Autodesk Inventor part; units mm, degrees
ref_plane "YZ Plane" through (0, 0, 0) normal (1, 0, 0) x (0, 1, 0)
ref_plane "XZ Plane" through (0, 0, 0) normal (0, 1, 0) x (-1, 0, 0)
ref_plane "XY Plane" through (0, 0, 0) normal (0, 0, 1) x (1, 0, 0)
sketch "Skizze1" plane through (0, 0, 0) normal (0, 0, 1) x (1, 0, 0)
  line L0 (-9.8619, 0) -> (59.1713, 0)
  line L1 (0, -1.8) -> (0, 10.8)
  line L2 (0, 0) -> (0, 9)
  line L3 (0, 9) -> (7, 9)
  line L4 (7, 9) -> (9.3094, 5)
  line L5 (9.3094, 5) -> (49.3094, 5)
  line L6 (49.3094, 5) -> (49.3094, 0)
  line L7 (49.3094, 0) -> (0, 0)
  dimension "d0" = 18
  dimension "d1" = 7
  dimension "d3" = 10
  dimension "d4" = 40
  dimension "d16" = 60
revolve "Umdrehung1" add sketch "Skizze1" angle 360 about axis through (-10, 0, 0) along (1, 0, 0)
chamfer "Fase1" distance 1 angle 45 1 edges at (49.3094, -5, 0)
chamfer "Fase2" distance 0.5 angle 45 1 edges at (0, -9, 0)
thread "Gewinde1"
sketch "Skizze2" plane through (0, 0, 0) normal (-1, 0, 0) x (0, 0, 1)
  spline S0 degree 3 poles (0.7512, 3.8741) (0.7506, 3.8768) (0.75, 3.8795) (0.7227, 3.995) (0.6691, 4.1023) (0.5302, 4.2738) (0.4382, 4.3487) (0.229, 4.4493) (0.1117, 4.475) (0, 4.475) knots 2.407009 2.407009 2.407009 2.407009 2.415407 2.415407 2.762565 2.762565 3.097556 3.097556 3.432546 3.432546 3.432546 3.432546
  spline S1 degree 3 poles (0, 4.475) (-0.1117, 4.475) (-0.229, 4.4493) (-0.4383, 4.3487) (-0.5302, 4.2739) (-0.6692, 4.1024) (-0.7228, 3.995) (-0.7501, 3.8795) (-0.7507, 3.8768) (-0.7514, 3.8741) knots 3.432546 3.432546 3.432546 3.432546 3.767537 3.767537 4.102528 4.102528 4.449685 4.449685 4.458083 4.458083 4.458083 4.458083
  spline S2 degree 3 poles (-0.7514, 3.8741) (-0.7825, 3.7367) (-0.83, 3.604) (-0.9596, 3.341) (-1.058, 3.1943) (-1.298, 2.9367) (-1.4398, 2.8257) (-1.7272, 2.6597) (-1.8942, 2.5924) (-2.2374, 2.5134) (-2.4136, 2.5016) (-2.7062, 2.5208) (-2.8448, 2.546) (-2.9794, 2.5877) knots 7.439135 7.439135 7.439135 7.439135 7.853901 7.853901 8.351764 8.351764 8.849626 8.849626 9.347489 9.347489 9.845351 9.845351 10.260117 10.260117 10.260117 10.260117
  spline S3 degree 3 poles (-2.9794, 2.5877) (-2.982, 2.5886) (-2.9847, 2.5894) (-3.0984, 2.6235) (-3.2181, 2.6307) (-3.4362, 2.5961) (-3.547, 2.5539) (-3.7387, 2.423) (-3.8196, 2.3342) (-3.8755, 2.2375) knots 2.407009 2.407009 2.407009 2.407009 2.415407 2.415407 2.762565 2.762565 3.097556 3.097556 3.432546 3.432546 3.432546 3.432546
  spline S4 degree 3 poles (-3.8755, 2.2375) (-3.9313, 2.1408) (-3.9677, 2.0263) (-3.9853, 1.7948) (-3.9664, 1.6777) (-3.8873, 1.4716) (-3.8212, 1.3716) (-3.7348, 1.2902) (-3.7328, 1.2882) (-3.7307, 1.2863) knots 3.432546 3.432546 3.432546 3.432546 3.767537 3.767537 4.102528 4.102528 4.449685 4.449685 4.458083 4.458083 4.458083 4.458083
  spline S5 degree 3 poles (-3.7307, 1.2863) (-3.6273, 1.1907) (-3.5361, 1.0832) (-3.3732, 0.8394) (-3.2953, 0.6809) (-3.1922, 0.3442) (-3.167, 0.1659) (-3.1669, -0.166) (-3.1921, -0.3443) (-3.2953, -0.681) (-3.3731, -0.8395) (-3.536, -1.0833) (-3.6272, -1.1908) (-3.7306, -1.2865) knots 7.439135 7.439135 7.439135 7.439135 7.853901 7.853901 8.351764 8.351764 8.849626 8.849626 9.347489 9.347489 9.845351 9.845351 10.260117 10.260117 10.260117 10.260117
  spline S6 degree 3 poles (-3.7306, -1.2865) (-3.7327, -1.2884) (-3.7347, -1.2903) (-3.8211, -1.3717) (-3.8872, -1.4717) (-3.9663, -1.6778) (-3.9852, -1.7948) (-3.9677, -2.0263) (-3.9313, -2.1408) (-3.8755, -2.2375) knots 2.407009 2.407009 2.407009 2.407009 2.415407 2.415407 2.762565 2.762565 3.097556 3.097556 3.432546 3.432546 3.432546 3.432546
  spline S7 degree 3 poles (-3.8755, -2.2375) (-3.8196, -2.3342) (-3.7387, -2.4229) (-3.547, -2.5539) (-3.4362, -2.5961) (-3.2182, -2.6306) (-3.0984, -2.6233) (-2.9848, -2.5893) (-2.9821, -2.5884) (-2.9794, -2.5876) knots 3.432546 3.432546 3.432546 3.432546 3.767537 3.767537 4.102528 4.102528 4.449685 4.449685 4.458083 4.458083 4.458083 4.458083
  spline S8 degree 3 poles (-2.9794, -2.5876) (-2.8449, -2.5459) (-2.7062, -2.5206) (-2.4136, -2.5014) (-2.2374, -2.5132) (-1.8942, -2.5923) (-1.7272, -2.6596) (-1.4397, -2.8256) (-1.2979, -2.9365) (-1.0578, -3.1942) (-0.9595, -3.3409) (-0.8298, -3.6039) (-0.7824, -3.7367) (-0.7512, -3.8741) knots 7.439135 7.439135 7.439135 7.439135 7.853901 7.853901 8.351764 8.351764 8.849626 8.849626 9.347489 9.347489 9.845351 9.845351 10.260117 10.260117 10.260117 10.260117
  spline S9 degree 3 poles (-0.7512, -3.8741) (-0.7506, -3.8768) (-0.75, -3.8795) (-0.7227, -3.995) (-0.6691, -4.1023) (-0.5302, -4.2738) (-0.4382, -4.3487) (-0.229, -4.4493) (-0.1117, -4.475) (0, -4.475) knots 2.407009 2.407009 2.407009 2.407009 2.415407 2.415407 2.762565 2.762565 3.097556 3.097556 3.432546 3.432546 3.432546 3.432546
  spline S10 degree 3 poles (0, -4.475) (0.1117, -4.475) (0.229, -4.4493) (0.4382, -4.3487) (0.5302, -4.2738) (0.6691, -4.1023) (0.7227, -3.995) (0.75, -3.8795) (0.7506, -3.8768) (0.7512, -3.8741) knots 3.432546 3.432546 3.432546 3.432546 3.767537 3.767537 4.102528 4.102528 4.449685 4.449685 4.458083 4.458083 4.458083 4.458083
  spline S11 degree 3 poles (0.7512, -3.8741) (0.7824, -3.7367) (0.8298, -3.604) (0.9595, -3.341) (1.0579, -3.1943) (1.2979, -2.9366) (1.4397, -2.8257) (1.7272, -2.6597) (1.8942, -2.5924) (2.2374, -2.5134) (2.4136, -2.5015) (2.7062, -2.5208) (2.8448, -2.546) (2.9794, -2.5877) knots 7.439135 7.439135 7.439135 7.439135 7.853901 7.853901 8.351764 8.351764 8.849626 8.849626 9.347489 9.347489 9.845351 9.845351 10.260117 10.260117 10.260117 10.260117
  spline S12 degree 3 poles (2.9794, -2.5877) (2.982, -2.5886) (2.9847, -2.5894) (3.0984, -2.6235) (3.2181, -2.6307) (3.4362, -2.5961) (3.547, -2.5539) (3.7387, -2.423) (3.8196, -2.3342) (3.8755, -2.2375) knots 2.407009 2.407009 2.407009 2.407009 2.415407 2.415407 2.762565 2.762565 3.097556 3.097556 3.432546 3.432546 3.432546 3.432546
  spline S13 degree 3 poles (3.8755, -2.2375) (3.9313, -2.1408) (3.9677, -2.0263) (3.9852, -1.7948) (3.9663, -1.6778) (3.8872, -1.4717) (3.8211, -1.3717) (3.7347, -1.2903) (3.7327, -1.2884) (3.7306, -1.2865) knots 3.432546 3.432546 3.432546 3.432546 3.767537 3.767537 4.102528 4.102528 4.449685 4.449685 4.458083 4.458083 4.458083 4.458083
  spline S14 degree 3 poles (3.7306, -1.2865) (3.6272, -1.1908) (3.536, -1.0833) (3.3731, -0.8395) (3.2953, -0.681) (3.1921, -0.3443) (3.1669, -0.166) (3.167, 0.1659) (3.1922, 0.3442) (3.2953, 0.6809) (3.3732, 0.8394) (3.5361, 1.0832) (3.6273, 1.1907) (3.7307, 1.2863) knots 7.439135 7.439135 7.439135 7.439135 7.853901 7.853901 8.351764 8.351764 8.849626 8.849626 9.347489 9.347489 9.845351 9.845351 10.260117 10.260117 10.260117 10.260117
  spline S15 degree 3 poles (3.7307, 1.2863) (3.7328, 1.2882) (3.7348, 1.2902) (3.8212, 1.3716) (3.8873, 1.4716) (3.9664, 1.6777) (3.9853, 1.7948) (3.9677, 2.0263) (3.9313, 2.1408) (3.8755, 2.2375) knots 2.407009 2.407009 2.407009 2.407009 2.415407 2.415407 2.762565 2.762565 3.097556 3.097556 3.432546 3.432546 3.432546 3.432546
  spline S16 degree 3 poles (3.8755, 2.2375) (3.8196, 2.3342) (3.7387, 2.423) (3.547, 2.5539) (3.4362, 2.5961) (3.2181, 2.6307) (3.0984, 2.6235) (2.9847, 2.5894) (2.982, 2.5886) (2.9794, 2.5877) knots 3.432546 3.432546 3.432546 3.432546 3.767537 3.767537 4.102528 4.102528 4.449685 4.449685 4.458083 4.458083 4.458083 4.458083
  spline S17 degree 3 poles (2.9794, 2.5877) (2.8448, 2.546) (2.7062, 2.5208) (2.4136, 2.5015) (2.2374, 2.5134) (1.8942, 2.5924) (1.7272, 2.6597) (1.4397, 2.8257) (1.2979, 2.9366) (1.0579, 3.1943) (0.9595, 3.341) (0.8298, 3.604) (0.7824, 3.7367) (0.7512, 3.8741) knots 7.439135 7.439135 7.439135 7.439135 7.853901 7.853901 8.351764 8.351764 8.849626 8.849626 9.347489 9.347489 9.845351 9.845351 10.260117 10.260117 10.260117 10.260117
  point P0 (0, 0)
  point P1 (0, 0)
  point P2 (0, 0)
extrude "Extrusion1" cut sketch "Skizze2" against normal blind 6
properties part number "Torx T50 M10 x 1,25" material "钢，高强度，低合金"
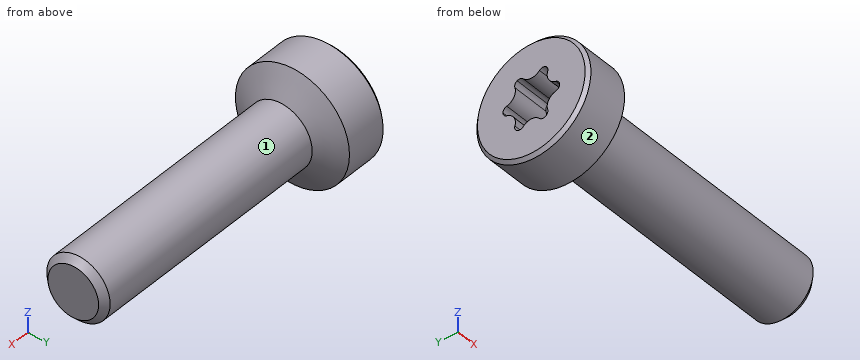
CAD build for the part. Positions are in the model's coordinates, mm. Face numbers are marked on the shaded views. A direction names the side the tool comes from. Give positions to 0.01 mm unless a question says otherwise; leave off trailing zeros. Write each loop counter-clockwise with the first axis right and the second up, starting at its lowest first coordinate (ties: lowest second). Pieces come first, ordered by that corner, then holes. Notation, with made-up numbers: M -36,60.5 L -24,60.5 A22 ccw -24,71.5 Z; hole C 33.25,-13 d8. An arc over 180 degrees is marked long. Return JSON: item names as keys, results as strings. Group by question number.
(1) Drill centre lines: L1, parallel to Z at x = 16, y = -4.25; L2, parallel to X at y = 0, z = 1; L3, parallel to Z at x = 38, y = 0. Where is each one in solid material? Low to high. Write a range as [from, to].
(2) Band-saw the part on A-A (x = 14). Give the cut face in (y, z).
(3) 3-axis set-ups, long thin cutter, end or side, ignore diameter. For the marked faces 1 and 2: which of +Z, -Z, +X, -X, +Y, -Y reach the whole face in a straight line?
(4) Flat gauge pins, fed straight in: pin 1 Ø8 at (x, z) = (14, -2) entering from -Y; pin 2 Ø5 at (x, y) = (37, -4) entering from +Z; pin 3 Ø1 at (x, y) = (22, -2.5) entering from -Z. Where does each tip first touch, or does it go through?
Entries:
{
 "1": {"L1": "z = [-2.63, 2.63]", "L2": "x = [6, 49.31]", "L3": "z = [-5, 5]"},
 "2": {"outline": "C 0,0 d10"},
 "3": {"face 1": "+X", "face 2": "+X, -X"},
 "4": {"pin 1": "stops at y = -5", "pin 2": "stops at z = 4.77", "pin 3": "stops at z = -4.58"}
}
